Input: part model. Units: mm. Frame: model coordinates. Face numbers are marked on the shaded views. A direction names the side the tool comes from. Give positions to 0.01 mm unless a question says otherwise; leave off trailing zeros. Loops run counter-clockwise (first coordinate to the right, second up) from the corner with the lowest first, then second, coordinate; pieces in that order, holes last. Notation, with made-up numbers: M -2,-3.5 L 57,-3.5 A15 cw 57,6.5 Z; hole C -31.75,1 d11. An arc over 180 degrees is marked long. Use a Markdown table: item, result. Add a question column.
from build123d import *

# Parameters (mm, degrees)
F0_R     = 25.446567
F1_DEPTH = 30


with BuildPart() as f1:
    # F0 (on Front) → F1 (new body)
    with BuildSketch(Plane.XZ):
        Polygon((60.751898, 31.746175), (-139.247308, 31.182794), (-139.247308, -18.817206), (-89.247308, -18.817206), (-113.978493, 0), (29.021507, 0), (10.751898, -18.253825), (60.751898, -18.253825), align=None)
        with BuildLine():
            Line((-95.085682, 107.776618), (-139.247308, 31.182794))
            Line((-139.247308, 31.182794), (60.751898, 31.746175))
            Line((60.751898, 31.746175), (5.600255, 105.301918))
            ThreePointArc((5.600255, 105.301918), (5.658245, 103.905416), (5.67758, 102.507845))
            ThreePointArc((5.67758, 102.507845), (-47.479786, 52.057386), (-95.085682, 107.776618))
        make_face()
        with BuildLine():
            ThreePointArc((5.600255, 105.301918), (-43.600489, 153.011972), (-95.085682, 107.776618))
            ThreePointArc((-95.085682, 107.776618), (-47.479786, 52.057386), (5.67758, 102.507845))
            ThreePointArc((5.67758, 102.507845), (5.658245, 103.905416), (5.600255, 105.301918))
        make_face()
        with Locations((-44.8418, 102.507845)):
            Circle(F0_R, mode=Mode.SUBTRACT)
    extrude(amount=F1_DEPTH)


solid = f1.part
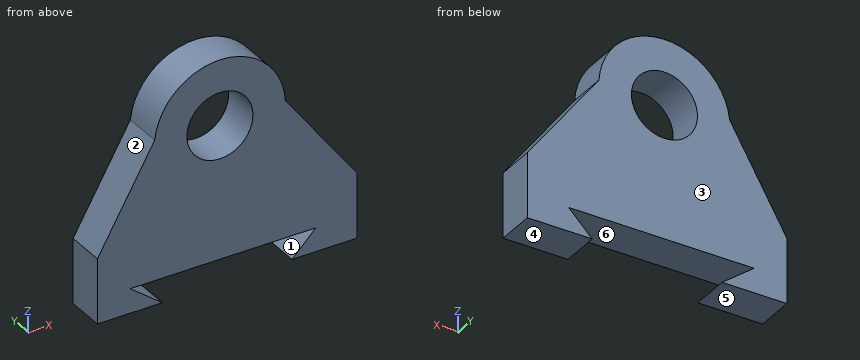
1) Reachability of the marked faces 4, 5 and 6 from +Z, -Z, +X, -X, +Y, -Y: full face, straight path, thin tool, end or side. Return the list, or none.
2) Section query D-D, the plane z = 67. Return the cut outline in (x, y), and give its area (3 significant figures).
3) Section query C-C, the plane y = -17.5. Return the cut outline in (x, z).
4) Contact query for flat-ended pins moving along their axis: P1, Ø1, axis at y = -8, z = 61, coming from the +X side; P2, Ø8, axis at x = 32, y = -22, coming from the +Z side; P3, Ø9, axis at x = -36.5, y = -8.5, coming from the -Z side. Output: stop coordinate, or through.
5) Ray query, line 1 (X direction, y = -18, z = 91.5); line 2 (X direction, y = -23.5, z = 82.5); line 3 (Z direction, x = -51, y = -20.25). Return the intervals inside material, ascending. Write a range as [from, to].
6) Section query A-A, the plane x = -91.5. Return the cut outline in (y, z), and give its area (3 significant figures).
7) Section query B-B, the plane z = 110. Return the cut outline in (x, y), and give its area (3 significant figures).
8) Pull-direction query (X, two-part tool) for the marked faces 1, 2 and 3; classes: pulls with the +X half, pulls with the -X half, needs draft (parallel to the pull), parting line crosses it, or undercut.
Entries:
| question | item | result |
|---|---|---|
| 1 | face 4 | -Z, +X, +Y, -Y |
| 1 | face 5 | -Z, +X, -X, +Y, -Y |
| 1 | face 6 | +Y, -Y |
| 2 | outline | M -118.6,-30 L 34.32,-30 L 34.32,0 L -118.6,0 Z |
| 2 | area | 4,590 mm² |
| 3 | outline | M -139.25,-18.82 L -89.25,-18.82 L -113.98,0 L 29.02,0 L 10.75,-18.25 L 60.75,-18.25 L 60.75,31.75 L 5.6,105.3 A50.52 ccw -95.09,107.78 L -139.25,31.18 Z; hole C -44.84,102.51 d50.89 |
| 4 | P1 | stops at x = 39.19 |
| 4 | P2 | stops at z = 75.43 |
| 4 | P3 | stops at z = 0 |
| 5 | line 1 | x = [-104.47, -67.78], [-21.9, 15.95] |
| 5 | line 2 | x = [-109.66, -60.56], [-29.12, 22.7] |
| 5 | line 3 | z = [0, 77.82], [127.2, 152.65] |
| 6 | outline | M -30,-18.82 L 0,-18.82 L 0,-17.1 L -30,-17.1 Z; M -30,0 L 0,0 L 0,121.88 L -30,121.88 Z |
| 6 | area | 3,710 mm² |
| 7 | outline | M -94.8,-30 L -69.16,-30 L -69.16,0 L -94.8,0 Z; M -20.52,-30 L 5.12,-30 L 5.12,0 L -20.52,0 Z |
| 7 | area | 1,540 mm² |
| 8 | face 1 | undercut |
| 8 | face 2 | pulls with the -X half |
| 8 | face 3 | needs draft |
